Autodesk Inventor part; units mm, degrees
ref_plane "YZ Plane" through (0, 0, 0) normal (1, 0, 0) x (0, 1, 0)
ref_plane "XZ Plane" through (0, 0, 0) normal (0, 1, 0) x (-1, 0, 0)
ref_plane "XY Plane" through (0, 0, 0) normal (0, 0, 1) x (1, 0, 0)
sketch "Sketch1" plane through (0, 0, 0) normal (0, 0, 1) x (1, 0, 0)
  line L0 (0, 10.9985) -> (9.525, -5.4993)
  line L1 (9.525, -5.4993) -> (-9.525, -5.4993)
  line L2 (-9.525, -5.4993) -> (0, 10.9985)
  line L3 (0, 4.8882) -> (4.2333, -2.4441)
  line L4 (4.2333, -2.4441) -> (-4.2333, -2.4441)
  line L5 (-4.2333, -2.4441) -> (0, 4.8882)
  point P0 (0, 0)
  point P1 (0, 0)
  point P2 (0, 0)
  dimension "d0" = 19.05
  dimension "d1" = 8.4667
extrude "Extrusion1" add sketch "Sketch1" against normal blind 16.9333
sketch "Sketch2" plane through (0, 0, -16.9333) normal (0, 0, -1) x (-1, 0, 0)
  circle A0 centre (0, 0) radius 6.35
  dimension "d4" = 12.7
extrude "Extrusion2" add sketch "Sketch2" along normal blind 8.4667
sketch "Sketch3" plane through (0, 0, -25.4) normal (0, 0, -1) x (-1, 0, 0)
  line L0 (4.4901, 0) -> (0, -4.4901)
  line L1 (0, -4.4901) -> (-4.4901, 0)
  line L2 (-4.4901, 0) -> (0, 4.4901)
  line L3 (0, 4.4901) -> (4.4901, 0)
  line L4 (4.4901, 0) -> (-4.4901, 0) construction
  line L5 (0, -4.4901) -> (0, 4.4901) construction
  point P0 (0, 0)
  dimension "d7" = 6.35
  dimension "d8" = 6.35
extrude "Extrusion3" cut sketch "Sketch3" against normal blind 6.35
properties part number "Driver Shaft Power" material "ABS Plastic"
CAD build for the part. Positions are in the model's coordinates, mm. A direction names the side the tool comes from. Round coordinates to 2 decimals unless told otherwise and drop trailing zeros. Write each loop counter-clockwise with the first axis right and the second up, starting at its lowest first coordinate (ties: lowest second). Pieces come first, ordered by that corner, then holes.
(1) Drop flat-ended pins along their axis: P1, Ø2.5, axis at x = 0, z = -8, coming from the +Y side; P2, Ø5, axis at y = 4, z = -5, coming from the -X side; P3, Ø6, axis at x = -1.5, y = 2, coming from the +Z side; P4, Ø1, axis at x = -5.5, y = 4, coming from the +Z side. Give the stop position or say it passes through.
(2) Slice it at B-B, the plane x = -2.5. Write the cut outline in (y, z), and give its area (3 significant figures).
(3) 3-axis set-ups, long thin cutter, end or side, ignore diameter. For faces 1 (the face through (-5, 3, -16.933)), 2 (the face through (0, -6, -16.933)), 3 (the face through (-2.146, 1.171, -8.348)): which of +Z, -Z, +X, -X, +Y, -Y reach the whole face in a straight line?
(4) Probe line 1 along Z through (x, y) = (6.75, -3.5); line 2 along Z through (x, y) = (0, 3.5); line 3 along Y through (x, z) = (-3, -12.5). List the from-to ranges inside material, lowest first.
(5) Mould opens along Y. For faces 4 (the face through (5, 3, -16.933)), 5 (the face through (-2.28, -2.21, -22.27)), 6 (the face through (-4.83, 2.63, -8.35)) say: pulls with the +Y half, pulls with the -Y half, needs draft (parallel to the pull), parting line crosses it, or undercut.
(6) Slice it at C-C, the plane y = -2. Write the cut outline in (x, z), and give its area (3 significant figures).
(7) Slice it at A-A, the plane z = -4.5. Write the cut outline in (x, y) (1 decimal).
(8) Slice it at D-D, the plane z = -23. Write the cut outline in (x, y).
From the geometry:
1. P1: stops at y = 11
1. P2: stops at x = -5.48
1. P3: stops at z = 0
1. P4: stops at z = -16.93
2. outline: (-5.84, -25.4) - (-1.99, -25.4) - (-1.99, -19.05) - (1.99, -19.05) - (1.99, -25.4) - (5.84, -25.4) - (5.84, -16.93) - (6.67, -16.93) - (6.67, 0) - (0.56, 0) - (0.56, -16.93) - (-2.44, -16.93) - (-2.44, 0) - (-5.5, 0) - (-5.5, -16.93) - (-5.84, -16.93) - close
2. area: 229 mm2
3. face 1: +Z, -X, +Y
3. face 2: +Z, +X, -X, -Y
3. face 3: +Z
4. line 1: z = -16.93 to 0
4. line 2: z = -19.05 to -16.93
4. line 3: y = -5.5 to -2.44, -0.31 to 5.8
5. face 4: needs draft
5. face 5: undercut
5. face 6: pulls with the +Y half
6. outline: (-7.5, -16.93) - (-6.03, -16.93) - (-6.03, -25.4) - (-2.49, -25.4) - (-2.49, -19.05) - (2.49, -19.05) - (2.49, -25.4) - (6.03, -25.4) - (6.03, -16.93) - (7.5, -16.93) - (7.5, 0) - (3.98, 0) - (3.98, -16.93) - (-3.98, -16.93) - (-3.98, 0) - (-7.5, 0) - close
6. area: 190 mm2
7. outline: (-9.5, -5.5) - (9.5, -5.5) - (0, 11) - close; hole (-4.2, -2.4) - (4.2, -2.4) - (0, 4.9) - close
8. outline: circle Ø12.7 at (0, 0); hole (-4.49, 0) - (0, -4.49) - (4.49, 0) - (0, 4.49) - close
